Here's how the part is built. I have some questions about the finished solid (model axes, mm). Face numbers are marked on the shaded views. A direction names the side the tool comes from. Give positions to 0.01 mm unless a question says otherwise; leave off trailing zeros. Loops run counter-clockwise (first coordinate to the right, second up) from the corner with the lowest first, then second, coordinate; pieces in that order, holes last. Notation, with made-up numbers: (48.25, 78) -> (96.25, 78) arc R20 ccw to (96.25, 90) -> close; hole circle Ø4 at (16.5, -6.5). An arc over 180 degrees is marked (long way). Answer in a Markdown table with one row per item. Add a question column.
Item 1: If we section it at D-D (y = 13): Write out the boundary of the cut face in (x, z).
Item 2: If we section it at A-A (z = 20): Write out the boundary of the cut face in (x, y), then the cut area to 3 significant figures.
Item 3: If we section it at B-B (z = 36): Write out the boundary of the cut face in (x, y), then the cut area to 3 significant figures.
Item 4: For P1, Ø4, axis at y = -53, z = 50.5, coming from the -X side; P2, Ø10, axis at x = -6, y = -29.5, coming from the +Z side; P3, Ø4, axis at y = -39.5, z = 50, coming from the +X side, each with a flat end and sliding along its axis, tell me the tip position at first contact or that it passes through.
Item 5: We'd pull the mould along Z, two halves only. Please class the marked faces 3, 4 and 5: released by +Z, released by -Z, zero draft, split by the parting line, or undercut.
Item 6: If I drill on line 1 (Z direction, x = 12.5, y = -60); line 2 (Y direction, x = 0.5, z = 17.5); line 3 (X direction, y = 7.5, z = 28), over which ranges is the centre line in solid material (lowest first)?
Item 7: Which directions (+Z, -Z, +X, -X, +Y, -Y) give clear straight access to the entire face, cutting with the end or side of a thin tool? Please do the marked faces 1 and 2.
Item 8: If we section it at C-C (x = 29): Write out the boundary of the cut face in (y, z).
Autodesk Fusion 360 part; units mm, degrees
sketch "Sketch1" plane through (0, 0, 0) normal (1, 0, 0) x (0, 1, 0)
  line L0 (-80, 0) -> (50, 0)
  line L1 (50, 0) -> (50, 60)
  line L2 (50, 60) -> (-80, 60)
  line L3 (-80, 60) -> (-80, 0)
  dimension "d1" = 130
  dimension "d2" = 60
extrude "Extrude1" add sketch "Sketch1" along normal blind 20
fillet "Fillet1" radius 20 2 edges at (10, -80, 60) (10, 50, 60)
sketch "Sketch2" plane through (20, 0, 0) normal (1, 0, 0) x (0, 1, 0)
  circle A0 centre (-60, 20) radius 10
  circle A1 centre (30, 20) radius 10
  arc A2 (50, 40) -> (30, 60) centre (30, 40) ccw
  line L0 (30, 60) -> (-60, 60)
  arc A3 (-60, 60) -> (-80, 40) centre (-60, 40) ccw
  line L1 (-80, 40) -> (-80, 0)
  line L2 (-80, 0) -> (50, 0)
  line L3 (50, 0) -> (50, 40)
  dimension "d11" = 20
  dimension "d14" = 90
  dimension "d15" = 0
extrude "Extrude2" cut sketch "Sketch2" against normal blind 20 contours A0 | A1
chamfer "Chamfer1" distance 1 angle 45 4 edges at (20, -69.3233, 23.6162) (20, 20.6767, 23.6162) (0, 20.6767, 16.3838) (0, -69.3233, 16.3838)
sketch "Sketch3" plane through (0, 0, 0) normal (-1, 0, 0) x (0, -1, 0)
  circle A0 centre (-30, 20) radius 11
  arc A1 (-30, 60) -> (-50, 40) centre (-30, 40) ccw
  line L0 (-50, 40) -> (-50, 0)
  line L1 (-50, 0) -> (80, 0)
  line L2 (80, 0) -> (80, 40)
  arc A2 (80, 40) -> (60, 60) centre (60, 40) ccw
  line L3 (60, 60) -> (-30, 60)
  circle A3 centre (60, 20) radius 11
  line L4 (-50, 0) -> (80, 0)
  line L5 (80, 0) -> (80, 2)
  line L6 (80, 2) -> (-50, 2)
  line L7 (-50, 2) -> (-50, 0)
  dimension "d19" = 2
extrude "Extrude3" add sketch "Sketch3" along normal blind 20 contours L0 L1 L2 L4 L5 L6 L7
extrude "Extrude4" add 1 faces at (-20, 6.6667, 0.6667) along direction (1, 0, 0) blind 60
fillet "Fillet4" radius 3 10 edges at (20, 50, 21) (20, 44.1421, 54.1421) (20, -15, 60) (20, -74.1421, 54.1421) (20, -80, 21) (0, 50, 21) (0, 44.1421, 54.1421) (0, -15, 60) (0, -74.1421, 54.1421) (0, -80, 21)
fillet "Fillet5" radius 1 6 edges at (40, -15, 2) (28.5, 50, 2) (28.5, -80, 2) (-8.5, 50, 2) (-20, -15, 2) (-8.5, -80, 2)
extrude "Extrude5" add 1 faces at (0, 6.6667, 0) along direction (0, 0, -1) blind 1
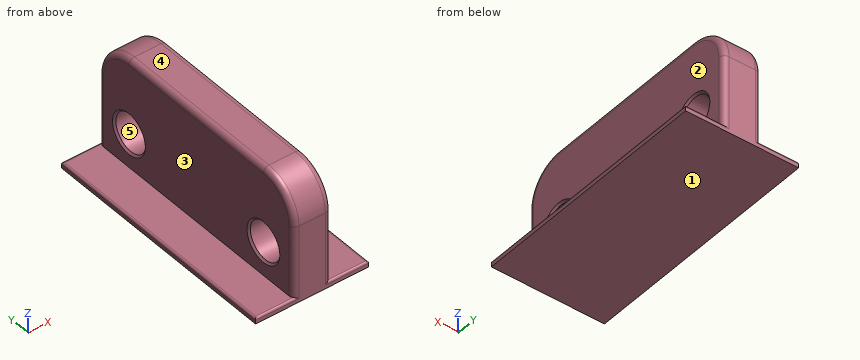
Recorded:
| question | item | result |
|---|---|---|
| 1 | outline | (-20, -1) -> (40, -1) -> (40, 1) arc R1 ccw to (39, 2) -> (20, 2) -> (20, 57) arc R3 ccw to (17, 60) -> (3, 60) arc R3 ccw to (0, 57) -> (0, 2) -> (-19, 2) arc R1 ccw to (-20, 1) -> close |
| 2 | outline | (0, -77) arc R3 ccw to (3, -80) -> (17, -80) arc R3 ccw to (20, -77) -> (20, -71) -> (19, -70) -> (1, -70) -> (0, -71) -> close; (0, -49) -> (1, -50) -> (19, -50) -> (20, -49) -> (20, 19) -> (19, 20) -> (1, 20) -> (0, 19) -> close; (0, 41) -> (1, 40) -> (19, 40) -> (20, 41) -> (20, 47) arc R3 ccw to (17, 50) -> (3, 50) arc R3 ccw to (0, 47) -> close |
| 2 | area | 1,790 mm^2 |
| 3 | outline | (0, -77) arc R3 ccw to (3, -80) -> (17, -80) arc R3 ccw to (20, -77) -> (20, 47) arc R3 ccw to (17, 50) -> (3, 50) arc R3 ccw to (0, 47) -> close |
| 3 | area | 2,590 mm^2 |
| 4 | P1 | stops at x = 0 |
| 4 | P2 | stops at z = 2 |
| 4 | P3 | stops at x = 20 |
| 5 | face 3 | zero draft |
| 5 | face 4 | released by +Z |
| 5 | face 5 | undercut |
| 6 | line 1 | z = -1 to 10, 30 to 60 |
| 6 | line 2 | y = -78.66 to -70.2, -49.8 to 19.8, 40.2 to 48.66 |
| 6 | line 3 | x = 0 to 20 |
| 7 | face 1 | -Z, +X, -X, +Y, -Y |
| 7 | face 2 | +Z, +X, +Y, -Y |
| 8 | outline | (-80, -1) -> (50, -1) -> (50, 1) arc R1 ccw to (49, 2) -> (-79, 2) arc R1 ccw to (-80, 1) -> close |
